Part model, mm, in its own coordinate system. Face numbers are marked on the shaded views. Coordinates: 2 decimals unless noted, no trailing zeros. Order: outer loops, then holes, each group sorted by start corner. A loop starts at its lowest first (then second) coordinate and runs counter-clockwise, first axis right, second up. Notation, with made-up numbers: (-40, 21.25) - (8, 21.25) arc R23 ccw to (8, 55.25) - close; hole circle Ø10 at (7.5, 14.25). An arc over 180 degrees is marked (long way). Use a Markdown table: item, result. Add a question column.
1) Two-plate mould, pull along Z, no slides. Class the marked faces 1, 2, 3 and 4: +Z half, -Z half, draft (parallel to the pull), parting line (faces both ways), or undercut.
2) Saw through at B-B on x = 0. Count the separate pieces of the cut face and the enclosed holes in it, then the cut area to 3 significant figures.
3) Saw through at A-A on y = 3.5. List the corners of the cut face in (x, z) (3 decimals), then the cut area to 3 significant figures.
4) Saw through at D-D on z = -3.5. List the corners of the cut face in (x, y) (3 decimals).
5) Saw through at C-C on z = 14. List the corners of the cut face in (x, y) (3 decimals), then the cut area to 3 significant figures.
6) Drop flat-ended pins along their axis: P1, Ø4, axis at y = 1, z = -5.5, coming from the -X side; P2, Ø1, axis at x = -7.5, y = 4, coming from the -Z side. Give the stop position or say it passes through.
7) Wall check: L1, parallel to Z at x = 0, y = 5.75 (3 decimals); L2, parallel to Z at x = -4.5, y = 5.5; L3, parallel to X at y = 2.75, z = 0 (3 decimals). Give the ranges that are in metal, low to high. Write a range as [from, to].
```python
from build123d import *

# Parameters (mm, degrees)
SKETCH1_R           = 9.525
SKETCH1_R_2         = 6.35
BOSS_EXTRUDE1_DEPTH = 9.525
BOSS_EXTRUDE2_DEPTH = 9.525
SKETCH3_R           = 3.175
CUT_EXTRUDE1_DEPTH  = 20.05


with BuildPart() as part:
    # Sketch1 → Boss-Extrude1 (new body)
    with BuildSketch(Plane(origin=(0, 0, 0), x_dir=(1, 0, 0), z_dir=(0, 1, 0))):
        Circle(SKETCH1_R)
        Circle(SKETCH1_R_2, mode=Mode.SUBTRACT)
    extrude(amount=BOSS_EXTRUDE1_DEPTH)

    # Sketch2 → Boss-Extrude2 (add, through all)
    with BuildSketch(Plane(origin=(0, 9.525, 0), x_dir=(1, 0, 0), z_dir=(0, 1, 0))):
        with BuildLine():
            Line((-9.525, 0), (-9.525, -21.100260413))
            Line((-9.525, -21.100260413), (9.525, -21.100260413))
            Line((9.525, -21.100260413), (9.525, 0))
            ThreePointArc((9.525, 0), (0, -9.525), (-9.525, 0))
        make_face()
    extrude(amount=-BOSS_EXTRUDE2_DEPTH)

    # Sketch3 → Cut-Extrude1 (cut, through all)
    with BuildSketch(Plane.ZY.offset(9.525)):
        with Locations((16.020260413, 4.7625)):
            Circle(SKETCH3_R)
    extrude(amount=-CUT_EXTRUDE1_DEPTH, mode=Mode.SUBTRACT)


solid = part.part
```
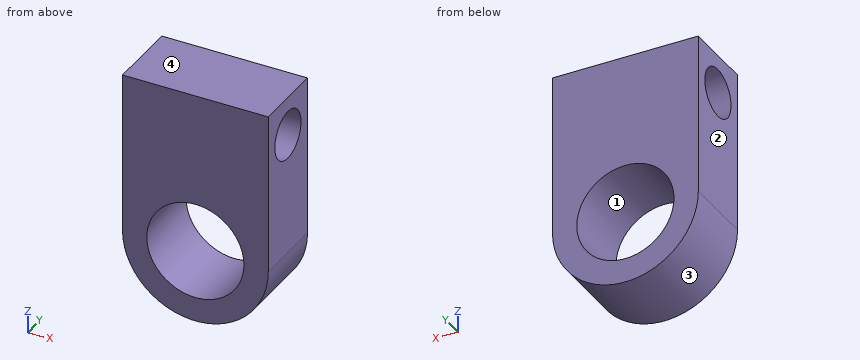
Results are:
| question | item | result |
|---|---|---|
| 1 | face 1 | undercut |
| 1 | face 2 | draft |
| 1 | face 3 | -Z half |
| 1 | face 4 | +Z half |
| 2 | separate pieces | 2 |
| 2 | enclosed holes | 1 |
| 2 | area | 139 mm2 |
| 3 | outline | (-9.525, 0) arc R9.525 ccw to (9.525, 0) - (9.525, 13.107) - (-9.525, 13.107) - close; (-9.525, 18.933) - (9.525, 18.933) - (9.525, 21.1) - (-9.525, 21.1) - close; hole circle Ø12.7 at (0, 0) |
| 3 | area | 307 mm2 |
| 4 | outline | (-8.859, 0) - (-5.298, 0) - (-5.298, 9.525) - (-8.859, 9.525) - close; (5.298, 0) - (8.859, 0) - (8.859, 9.525) - (5.298, 9.525) - close |
| 5 | outline | (-9.525, 0) - (9.525, 0) - (9.525, 2.313) - (-9.525, 2.313) - close; (-9.525, 7.212) - (9.525, 7.212) - (9.525, 9.525) - (-9.525, 9.525) - close |
| 5 | area | 88.1 mm2 |
| 6 | P1 | x = -8.86 |
| 6 | P2 | z = -6.46 |
| 7 | L1 | [-9.525, -6.35], [6.35, 13.003], [19.038, 21.1] |
| 7 | L2 | [-8.39, -4.48], [4.48, 12.93], [19.11, 21.1] |
| 7 | L3 | [-9.525, -6.35], [6.35, 9.525] |
